Part model, mm, in its own coordinate system. A direction names the side the tool comes from. Coordinates: 2 decimals unless noted, no trailing zeros. Write each loop counter-clockwise with the first axis right and the second up, starting at its lowest first coordinate (ties: lowest second). Pieces come first, ordered by that corner, then holes. Notation, with made-up numbers: (54, 71.5) - (87, 71.5) arc R12 cw to (87, 86.5) - close; hole circle Ø6 at (1.5, 89). An arc over 180 degrees is marked (long way). Use a Markdown table: item, result.
Autodesk Inventor part; units mm, degrees
ref_plane "YZ Plane" through (0, 0, 0) normal (1, 0, 0) x (0, 1, 0)
ref_plane "XZ Plane" through (0, 0, 0) normal (0, 1, 0) x (-1, 0, 0)
ref_plane "XY Plane" through (0, 0, 0) normal (0, 0, 1) x (1, 0, 0)
sketch "Sketch1" plane through (0, 0, 0) normal (1, 0, 0) x (0, 1, 0)
  circle A0 centre (0, 0) radius 17.5
  dimension "d0" = 35
extrude "Extrusion1" add sketch "Sketch1" along normal blind 5
sketch "Sketch2" plane through (5, 0, 0) normal (1, 0, 0) x (0, 0, -1)
  circle A0 centre (0, 0) radius 3
  dimension "d3" = 6
extrude "Extrusion2" add sketch "Sketch2" against normal blind 9
sketch "Sketch3" plane through (-4, 0, 0) normal (-1, 0, 0) x (0, 0, 1)
  circle A0 centre (0, 0) radius 1.5
  dimension "d6" = 3
extrude "Extrusion3" cut sketch "Sketch3" against normal blind 4
properties part number "Front Wheel" material "PC/ABS Plastic"
Item 1: Drill centre lines: probe 1 along Y at (x, z) = (-1.95, 0); probe 2 along X at (y, z) = (12, 11); probe 3 along Z at (x, y) = (0.5, -9.5). Where is each one in solid material? Low to high.
From the geometry:
| item | result |
|---|---|
| probe 1 | -3 to -1.5, 1.5 to 3 |
| probe 2 | 0 to 5 |
| probe 3 | -14.7 to 14.7 |
Item 2: Drop flat-ended pins along their axis: P1, Ø10.5, axis at y = 7.5, z = 4, coming from the -X side; P2, Ø1.5, axis at x = 3.5, y = 4, coming from the -Z side; P3, Ø5, axis at x = 1.5, y = 11, coming from the +Z side. Give the stop position or say it passes through.
From the geometry:
| item | result |
|---|---|
| P1 | x = 0 |
| P2 | z = -17.2 |
| P3 | z = 15.3 |
Item 3: Band-saw the part on D-D, the plane x = 3.25. Give the cut face in (y, z).
From the geometry:
| item | result |
|---|---|
| outline | circle Ø35 at (0, 0) |
Item 4: Which spindle directions (+Z, -Z, +X, -X, +Y, -Y) get a long thin tool onto all of the face, cutting with end or side? Do faces 1 (the face through (2.465, -13.887, 10.648)), 2 (the face through (-2.03, 0.07, -1.5)). Say none if no direction does.
From the geometry:
| item | result |
|---|---|
| face 1 | +X, -X |
| face 2 | -X |
Item 5: Band-saw the part on C-C, the plane x = -0.75. Give the cut face in (y, z), then the cut area to 3 significant figures.
From the geometry:
| item | result |
|---|---|
| outline | circle Ø6 at (0, 0); hole circle Ø3 at (0, 0) |
| area | 21.2 mm^2 |
Item 6: Two-plate mould, pull along Z, no slides. Class faces 3 (the face through (5, 0, 0)), 4 (the face through (-2, 0, 3)), 5 (the face through (0, 0, 0)): pulls with the +Z half, pulls with the -Z half, needs draft (parallel to the pull), parting line crosses it, or undercut.
From the geometry:
| item | result |
|---|---|
| face 3 | needs draft |
| face 4 | parting line crosses it |
| face 5 | undercut |
Item 7: Band-saw the part on A-A, the plane z = 0. Give the cut face in (x, y).
From the geometry:
| item | result |
|---|---|
| outline | (-4, -3) - (0, -3) - (0, -17.5) - (5, -17.5) - (5, 17.5) - (0, 17.5) - (0, 3) - (-4, 3) - (-4, 1.5) - (0, 1.5) - (0, -1.5) - (-4, -1.5) - close |
